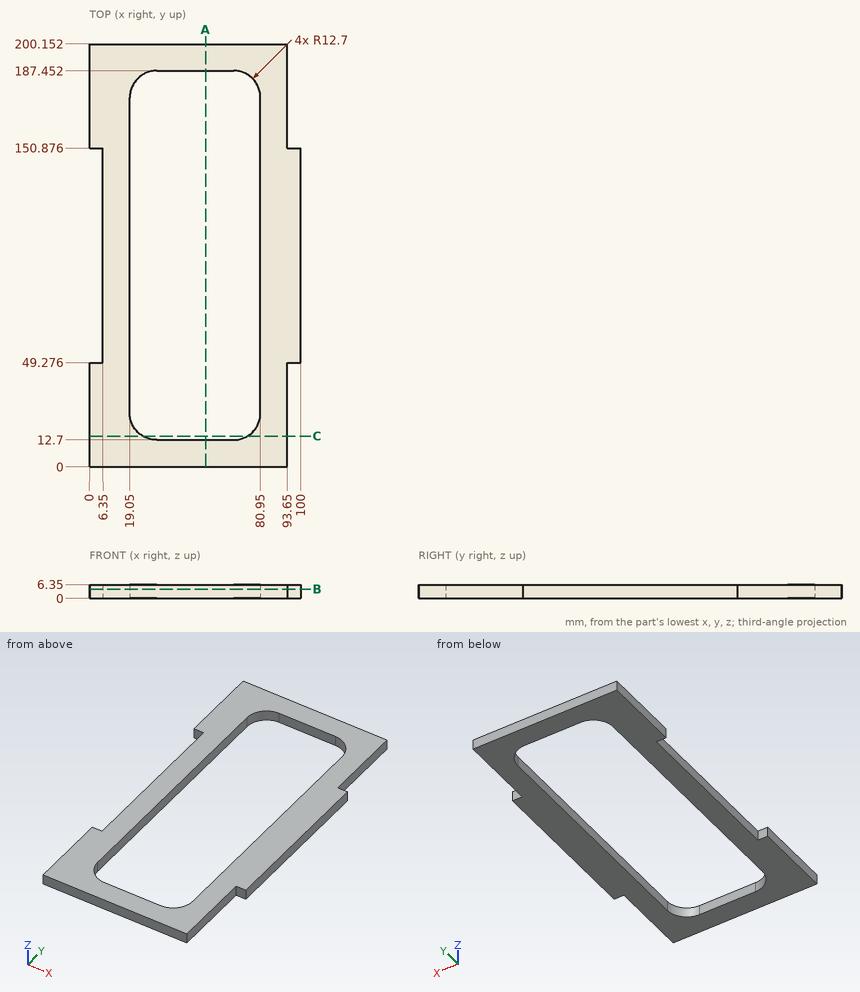
Geometry check sheet. Reference: drawing and pictorial views, mm from the part's lowest x, y, z. Give positions to 0.01 mm unless a question says otherwise; leave off trailing zeros. Write each loop counter-clockwise with the first axis right and the second up, starting at its lowest first coordinate (ties: lowest second). Pieces come first, ordered by that corner, then holes.
Item 1: Cross-section at B-B (z = 4.25). Enter the section's corners in (x, y), and give its area (3 significant figures).
Item 2: Cross-section at C-C (y = 14.5). Enter the section's corners in (x, z).
Item 3: Cross-section at A-A (x = 55). Enter the section's corners in (y, z).
Item 4: Gauge pin test, flat end, axial feed: pin 1 (3 mm diameter, centred on y = 87, z = 2, fed in from -X). Record the tip position at first contact, or that the pin passes through.
Item 5: Scan lines: L1, parallel to X at y = 28.5, z = 4.5; L2, parallel to X at y = 105, z = 2; L3, parallel to Y at x = 51, z = 1.75. Record each from-to range of solid material in increasing order.
Report:
1. outline: (0, 0) - (93.65, 0) - (93.65, 49.28) - (100, 49.28) - (100, 150.88) - (93.65, 150.88) - (93.65, 200.15) - (0, 200.15) - (0, 150.88) - (6.35, 150.88) - (6.35, 49.28) - (0, 49.28) - close; hole (19.05, 25.4) arc R12.7 ccw to (31.75, 12.7) - (68.25, 12.7) arc R12.7 ccw to (80.95, 25.4) - (80.95, 174.75) arc R12.7 ccw to (68.25, 187.45) - (31.75, 187.45) arc R12.7 ccw to (19.05, 174.75) - close
1. area: 8,070 mm2
2. outline: (0, 0) - (25.23, 0) - (25.23, 6.35) - (0, 6.35) - close; (74.77, 0) - (93.65, 0) - (93.65, 6.35) - (74.77, 6.35) - close
3. outline: (0, 0) - (12.7, 0) - (12.7, 6.35) - (0, 6.35) - close; (187.45, 0) - (200.15, 0) - (200.15, 6.35) - (187.45, 6.35) - close
4. pin 1: stops at x = 6.35
5. L1: x = 0 to 19.05, 80.95 to 93.65
5. L2: x = 6.35 to 19.05, 80.95 to 100
5. L3: y = 0 to 12.7, 187.45 to 200.15
